Input: part model. Units: mm. Frame: model coordinates. Give positions to 0.01 mm unless a question says otherwise; leave off trailing zeros. Order: outer loops, then holes, each group sorted by start corner. A loop starts at its lowest first (then second) coordinate and runs counter-clockwise, first axis right, second up. Notation, with made-up numbers: M 69.5,3.25 L 90.5,3.25 A22 ccw 90.5,36.25 Z; hole C -12,33 d5. An arc over 180 degrees is marked long. Use a Markdown table: item, result.
from build123d import *

# Parameters (mm, degrees)
SKETCH1_W            = 150
SKETCH1_H            = 74.66
BASE_FLANGE1_DEPTH   = 1.75
CUT_EXTRUDE1_REACH   = 107.84
SKETCH2_W            = 40
SKETCH2_H            = 10
M3_CLEARANCE_HOLE1_D = 3.4
FILLET1_R            = 3.175


# Sheet-metal steps are written as plain solids
with BuildPart() as part:
    # Sketch1 → Base-Flange1 (new body)
    with BuildSketch(Plane.XY):
        with Locations((0, 37.33)):
            Rectangle(SKETCH1_W, SKETCH1_H)
    extrude(amount=-BASE_FLANGE1_DEPTH)

    # Sketch2 → Cut-Extrude1 (cut, up to next)
    with BuildSketch(Plane.XY, mode=Mode.PRIVATE) as cut_extrude1_sk1:
        with Locations((0, 5)):
            Rectangle(SKETCH2_W, SKETCH2_H)
    cut_extrude1_tool1 = extrude(cut_extrude1_sk1.sketch, amount=-CUT_EXTRUDE1_REACH, mode=Mode.PRIVATE) & part.part
    add(cut_extrude1_tool1.solids().sort_by_distance((0, 5, 0))[0], mode=Mode.SUBTRACT)

    # M3 Clearance Hole1 (through all)
    with Locations(Plane.XY):
        with Locations((63.325, 68.66), (63.325, 7.125)):
            m3_clearance_hole1 = Hole(M3_CLEARANCE_HOLE1_D / 2)

    # Mirror1: M3 Clearance Hole1 across plane
    add(m3_clearance_hole1.mirror(Plane(origin=(0, 0, 0), x_dir=(0, 0, 1), z_dir=(1, 0, 0))), mode=Mode.SUBTRACT)

    # Fillet1
    fillet1_edges = [part.edges().sort_by_distance(p)[0] for p in [
        (75, 0, -0.875),
        (-75, 0, -0.875),
    ]]
    fillet(fillet1_edges, radius=FILLET1_R)


solid = part.part
1) Mould query, pull axis Y, two halves, no side actions, for faces 1 (the face through (-65.023, 7.2, -0.887)), 2 (the face through (-74.09, 0.95, -0.89)), 3 (the face through (-1, 38, 0)). Classes: released by +Y, released by -Y, zero draft, split by the parting line, or undercut.
Response values:
| item | result |
|---|---|
| face 1 | undercut |
| face 2 | released by -Y |
| face 3 | zero draft |
2) Cut plane B-B on z = -1.35. Return loops of the section in (x, y) (3 decimals), and give its area (3 significant figures).
Response values:
| item | result |
|---|---|
| outline | M -75,3.175 A3.175 ccw -71.825,0 L -20,0 L -20,10 L 20,10 L 20,0 L 71.825,0 A3.175 ccw 75,3.175 L 75,74.66 L -75,74.66 Z; hole C -63.325,7.125 d3.4; hole C -63.325,68.66 d3.4; hole C 63.325,7.125 d3.4; hole C 63.325,68.66 d3.4 |
| area | 10,800 mm² |
3) First-contact query: pin 1 Ø3 at (x, y) = (63.325, 7.125) entering from +Z; pin 2 Ø0.9 at (x, z) = (6, -1) entering from -Y. Flat tips, straight axial feed; report the tip coordinate or a pass-through.
Response values:
| item | result |
|---|---|
| pin 1 | passes through |
| pin 2 | stops at y = 10 |
4) Cut plane A-A on y = 68.66. Return loops of the section in (x, z) (3 decimals).
Response values:
| item | result |
|---|---|
| outline | M -75,-1.75 L -65.025,-1.75 L -65.025,0 L -75,0 Z; M -61.625,-1.75 L 61.625,-1.75 L 61.625,0 L -61.625,0 Z; M 65.025,-1.75 L 75,-1.75 L 75,0 L 65.025,0 Z |
5) Material intervals for line 1 (X direction, y = 68.66, z = -0.95) (3 decimals); line 2 (X direction, y = 4, z = -0.85); line 3 (Y direction, x = -2.5, z = -1), sorted ascending. Write a range as from..to.
Response values:
| item | result |
|---|---|
| line 1 | x = -75..-65.025, -61.625..61.625, 65.025..75 |
| line 2 | x = -75..-20, 20..75 |
| line 3 | y = 10..74.66 |
6) Cut plane C-C on x = 7. Return loops of the section in (y, z), and give its area (3 significant figures).
Response values:
| item | result |
|---|---|
| outline | M 10,-1.75 L 74.66,-1.75 L 74.66,0 L 10,0 Z |
| area | 113 mm² |
